```python
from build123d import *

# Parameters (mm, degrees)
F_10_5_10_5_DIAMETER_HOLE1_D     = 10.5
F_10_5_10_5_DIAMETER_HOLE1_DEPTH = 35
F_10_5_10_5_DIAMETER_HOLE1_TIP   = 3.15451825


with BuildPart() as part:
    # Sketch1 → Revolve1 (revolve)
    with BuildSketch(Plane.XY, mode=Mode.PRIVATE) as revolve1_sk:
        Polygon((-32.34392041, -25), (-12.34392041, -25), (-12.34392041, -26.5), (77.65607959, -26.5), (77.65607959, -27.5), (82.65607959, -27.5), (82.65607959, -25), (477.65607959, -25), (477.65607959, 0), (-32.34392041, 0), align=None)
    revolve(revolve1_sk.sketch.rotate(Axis((477.65607959, 0, 0), (-1, 0, 0)), 270), axis=Axis((477.65607959, 0, 0), (-1, 0, 0)))

    # Ø10.5 (10.5) Diameter Hole1
    with Locations(Plane(origin=(477.65607959, 0, 0), x_dir=(0, 0, 1), z_dir=(1, 0, 0))):
        with Locations((0, 0)):
            Hole(F_10_5_10_5_DIAMETER_HOLE1_D / 2, depth=F_10_5_10_5_DIAMETER_HOLE1_DEPTH)
            with Locations((0, 0, -(F_10_5_10_5_DIAMETER_HOLE1_DEPTH + F_10_5_10_5_DIAMETER_HOLE1_TIP / 2))):  # 118° drill point
                Cone(0, F_10_5_10_5_DIAMETER_HOLE1_D / 2, F_10_5_10_5_DIAMETER_HOLE1_TIP, mode=Mode.SUBTRACT)


solid = part.part
```
The model under review builds one solid part; all positions refer to its coordinate system, in mm. A direction names the side the tool comes from. Coordinates: 2 decimals unless noted, no trailing zeros. Write each loop counter-clockwise with the first axis right and the second up, starting at its lowest first coordinate (ties: lowest second). Pieces come first, ordered by that corner, then holes. Notation, with made-up numbers: (57.5, 38) - (87.5, 38) arc R23 cw to (87.5, 71) - close; hole circle Ø6 at (32.5, 68). An arc over 180 degrees is marked (long way). Answer in a Markdown table with one row per item. Add a question column.
Q1. To check wall thickness, follow line 1 along Y through (x, z) = (460, 0); line 2 along X through (y, z) = (25, 9); line 3 along X through (y, z) = (25.5, 4.5). State the ranges of each line that lie inside material, in increasing order. Write a range as from..to.
Q2. Consider section C-C on y = -10. Give the boundary of the cut face in (x, z).
Q3. Clearance check with flat-ended pins moving along their axes: pin 1 (1.5 mm diameter, centred on x = 262, y = 14, fed in from -Z); pin 2 (6 mm diameter, centred on x = 413, z = -10, fed in from -Y); pin 3 (5 mm diameter, centred on x = 333.5, z = 15, fed in from +Y). State where each tip first meets the part, or that it passes through.
Q4. Consider section B-B on x = 71.5. Give the boundary of the cut face in (y, z), then the cut area to 3 significant figures.
Q5. Consider section A-A on z = -18. Give the boundary of the cut face in (x, y).
Q6. Consider section D-D on x = 136. Give the boundary of the cut face in (y, z), then the cut area to 3 significant figures.
Q7. For faces 4 (the face through (-12.344, -16, 20)), 5 (the face through (82.656, 22.3, -12.1)), 6 (the face through (477.656, -6, 0)), list the 3-axis set-ups (+Z, -Z, +X, -X, +Y, -Y) from which the entire face can be reached by the end or side of a thin tool; tool diameter is ignored.
Q8. Draft analysis for pull direction Z (two halves, no side actions). For faces 1 (the face through (282.921, -7.509, -23.846)), 2 (the face through (459.9, -1.6, -5)), 3 (the face through (-32.344, 0, 0)), state which applies: +Z half, -Z half, draft (parallel to the pull), parting line (faces both ways), or undercut.
Answers below:
| question | item | result |
|---|---|---|
| 1 | line 1 | -25..-5.25, 5.25..25 |
| 1 | line 2 | 77.66..82.66 |
| 1 | line 3 | -12.34..82.66 |
| 2 | outline | (-32.34, -22.91) - (-12.34, -22.91) - (-12.34, -24.54) - (77.66, -24.54) - (77.66, -25.62) - (82.66, -25.62) - (82.66, -22.91) - (477.66, -22.91) - (477.66, 22.91) - (82.66, 22.91) - (82.66, 25.62) - (77.66, 25.62) - (77.66, 24.54) - (-12.34, 24.54) - (-12.34, 22.91) - (-32.34, 22.91) - close |
| 3 | pin 1 | z = -21.2 |
| 3 | pin 2 | y = -24 |
| 3 | pin 3 | y = 21.65 |
| 4 | outline | circle Ø53 at (0, 0) |
| 4 | area | 2,210 mm² |
| 5 | outline | (-32.34, -17.35) - (-12.34, -17.35) - (-12.34, -19.45) - (77.66, -19.45) - (77.66, -20.79) - (82.66, -20.79) - (82.66, -17.35) - (477.66, -17.35) - (477.66, 17.35) - (82.66, 17.35) - (82.66, 20.79) - (77.66, 20.79) - (77.66, 19.45) - (-12.34, 19.45) - (-12.34, 17.35) - (-32.34, 17.35) - close |
| 6 | outline | circle Ø50 at (0, 0) |
| 6 | area | 1,960 mm² |
| 7 | face 4 | -X |
| 7 | face 5 | +X |
| 7 | face 6 | +Z, -Z, +X, +Y, -Y |
| 8 | face 1 | parting line |
| 8 | face 2 | undercut |
| 8 | face 3 | draft |
